```python
from build123d import *

# Parameters (mm, degrees)
F0_R     = 1.5875
F1_DEPTH = 3.175


with BuildPart() as f1:
    # F0 (on Right) → F1 (new body)
    with BuildSketch(Plane.YZ):
        Polygon((-30.874995, 25.4), (-30.874995, 0), (-24.04999, 0), (-24.04999, 12.7), (-1.82499, 12.7), (-1.82499, 0), (30.874995, 0), (30.874995, 6.35), (30.874995, 25.4), align=None)
        with Locations((6.825005, 6.35)):
            Circle(F0_R, mode=Mode.SUBTRACT)
    extrude(amount=F1_DEPTH)


solid = f1.part
```
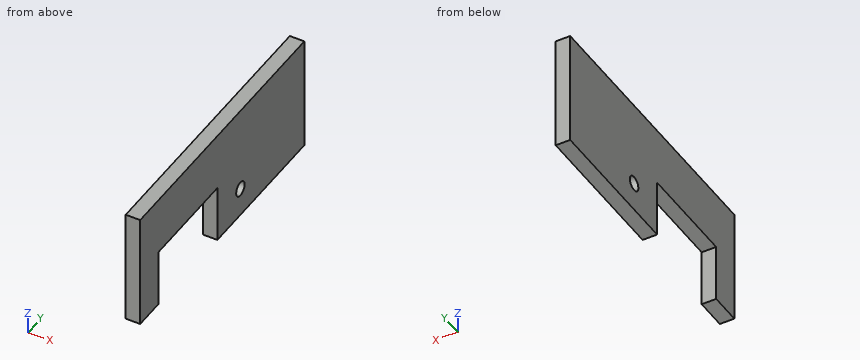
For this review, take the finished solid that the model builds, in its own axes (mm). Round coordinates to 2 decimals unless told otherwise and drop trailing zeros. Write each loop counter-clockwise with the first axis right and the second up, starting at its lowest first coordinate (ties: lowest second). Pieces come first, ordered by that corner, then holes. Notation, with made-up numbers: (40, 87.5) - (75, 87.5) arc R10 ccw to (75, 94.5) - close; hole circle Ø4 at (-17.75, 41). An arc over 180 degrees is marked (long way). Answer as CSV lines item,"result". Start each with the question number.
(1) Add section C-C, the plane z = 3. State the section outline as (x, y) points (3 decimals), plus the area to 3 significant figures.
(2) For pin 1 (2.5 mm diameter, centred on y = 6.83, z = 6.35, fed in from +X); pin 2 (1.6 mm diameter, centred on x = 2.5, y = -15, fed in from -Z), all flat-tipped, find the tip position at first contact; note any pin that passes through.
(3) Add section D-D, the plane y = -16. State the section outline as (x, z) points (3 decimals), plus the area to 3 significant figures.
(4) Add section B-B, the plane z = 6.35. State how many separate pieces and enclosed holes the cut face has, plus the area to 3 significant figures.
(5) For line 1 (Y direction, x = 0.95, z = 4) (3 decimals); line 2 (Y direction, x = 0.85, z = 5.5) (3 decimals); line 3 (Y direction, x = 2.75, z = 7.25) (3 decimals), list the stretches that pass through material, from the lowest coordinate up.
From the geometry:
1,outline,"(0, -30.875) - (3.175, -30.875) - (3.175, -24.05) - (0, -24.05) - close; (0, -1.825) - (3.175, -1.825) - (3.175, 30.875) - (0, 30.875) - close"
1,area,"125 mm²"
2,pin 1,"passes through"
2,pin 2,"stops at z = 12.7"
3,outline,"(0, 12.7) - (3.175, 12.7) - (3.175, 25.4) - (0, 25.4) - close"
3,area,"40.3 mm²"
4,separate pieces,"3"
4,enclosed holes,"0"
4,area,"115 mm²"
5,line 1,"y = -30.875 to -24.05, -1.825 to 30.875"
5,line 2,"y = -30.875 to -24.05, -1.825 to 5.484, 8.166 to 30.875"
5,line 3,"y = -30.875 to -24.05, -1.825 to 5.517, 8.133 to 30.875"
